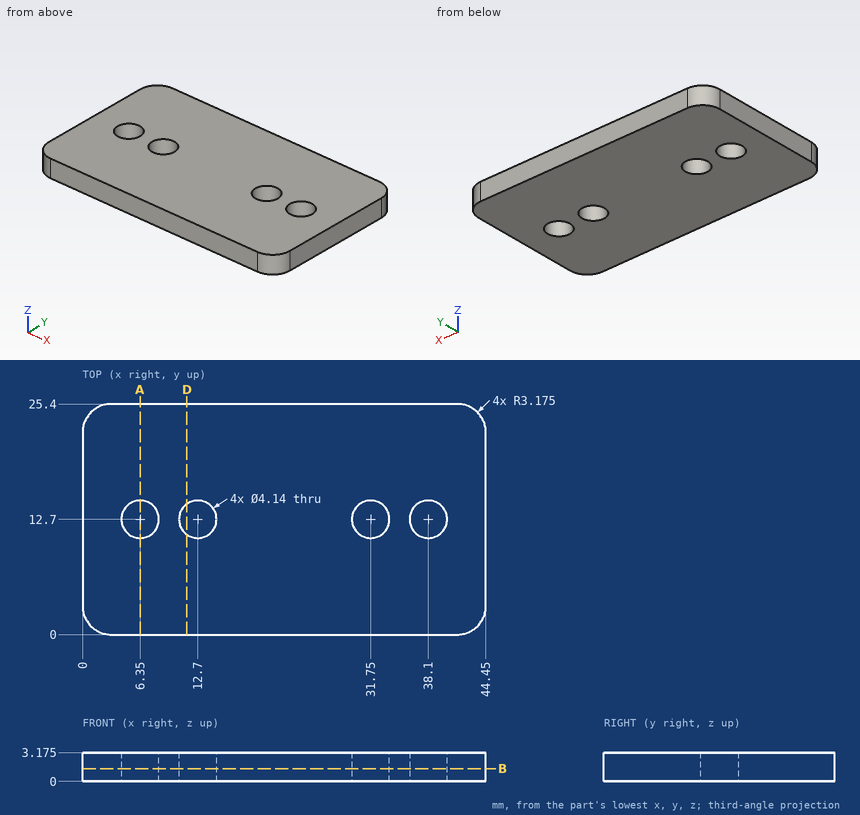
For this review, use the dimensioned drawing (mm, ordinates from the lowest corner) and the shaded views. Round coordinates to 2 decimals unless told otherwise and drop trailing zeros. Write each loop counter-clockwise with the first axis right and the second up, starting at its lowest first coordinate (ties: lowest second). Pieces come first, ordered by that corner, then holes. Notation, with made-up numbers: (50.25, -38) -> (108.25, -38) arc R22 ccw to (108.25, -12) -> close; hole circle Ø7 at (70, 34.25). An arc over 180 degrees is marked (long way). Use CSV: the item, a comma, the result in double quotes.
(1) Clearance check with a flat-ended pin moving along its axis: P1, Ø2.5, axis at x = 6.35, y = 12.7, coming from the -Z side. State where the tip first meets the part, or that it passes through.
Computed values:
P1,"through"
(2) Consider section B-B, the plane z = 1.4. Give the number of separate pieces and of enclosed holes in the cut face, plus the area to 3 significant figures.
Computed values:
separate pieces,"1"
enclosed holes,"4"
area,"1,070 mm²"
(3) Consider section A-A, the plane x = 6.35. Give the boundary of the cut face in (y, z) (1 decimal), plus the area to 3 significant figures.
Computed values:
outline,"(0, 0) -> (10.6, 0) -> (10.6, 3.2) -> (0, 3.2) -> close; (14.8, 0) -> (25.4, 0) -> (25.4, 3.2) -> (14.8, 3.2) -> close"
area,"67.5 mm²"
(4) To check wall thickness, follow L1, parallel to X at y = 12.5, z = 0.25; L2, parallel to Y at x = 12.7, z = 0.85; L3, parallel to X at y = 13, z = 0.5. State the ranges of each line that lie inside material, in increasing order. Write a range as [from, to].
Computed values:
L1,"[0, 4.29], [8.41, 10.64], [14.76, 29.69], [33.81, 36.04], [40.16, 44.45]"
L2,"[0, 10.63], [14.77, 25.4]"
L3,"[0, 4.3], [8.4, 10.65], [14.75, 29.7], [33.8, 36.05], [40.15, 44.45]"
(5) Consider section D-D, the plane x = 11.5. Give the boundary of the cut face in (y, z) (1 decimal).
Computed values:
outline,"(0, 0) -> (11, 0) -> (11, 3.2) -> (0, 3.2) -> close; (14.4, 0) -> (25.4, 0) -> (25.4, 3.2) -> (14.4, 3.2) -> close"
